Model file for the job. Use its own axes, mm. A direction names the side the tool comes from. Give positions to 0.01 mm unless a question says otherwise; leave off trailing zeros. Write each loop counter-clockwise with the first axis right and the second up, starting at its lowest first coordinate (ties: lowest second). Pieces come first, ordered by that corner, then holes. Notation, with made-up numbers: (30, -14.5) - (81, -14.5) arc R15 cw to (81, 3.5) - close; hole circle Ø8 at (56, 69.25). An arc over 180 degrees is marked (long way). One line per item, written item: value. Start each with the question number.
(1) 3-axis set-ups, long thin cutter, end or side, ignore diameter. For faces 1 (the face through (-3, -3, 11.176)), 2 (the face through (5, 2, 0)): which of +Z, -Z, +X, -X, +Y, -Y reach the whole face in a straight line?
(2) Drop flat-ended pins along their axis: P1, Ø1.5, axis at y = 0.5, z = 9, coming from the -X side; P2, Ø1, axis at y = 2, z = 4, coming from the -X side; P3, Ø2, axis at x = -2.5, z = 10, coming from the +Y side. Give the stop position or say it passes through.
(3) Cut at D-D, the plane z = 2.75. List the corners of the cut face in (x, y), and give its area (3 significant figures).
(4) Cut at C-C, the plane y = -4.75. List the corners of the cut face in (x, z), and give its area (3 significant figures).
(5) Mould opens along Y. For faces 3 (the face through (0.9, -3.9, -0.9)), 4 (the face through (-3, -3, -1.778)), 5 (the face through (-0.661, 5.037, 5.51)), 6 (the face through (-0.86, -3.874, 5.51)) say: pulls with the +Y half, pulls with the -Y half, needs draft (parallel to the pull), parting line crosses it, or undercut.
(6) Probe L1, parallel to Y at x = 0, z = 7; L2, parallel to Y at x = 0, z = -1.1; L3, parallel to Z at x = 4, y = 4.75. List the from-to ranges inside material, lowest first.
from build123d import *

# Parameters (mm, degrees)
SKETCH1_R      = 5.08
SKETCH1_R_2    = 3.96875
EXTRUDE1_DEPTH = 11.176
SKETCH2_R      = 7.112
SKETCH2_R_2    = 4.0005
EXTRUDE2_DEPTH = 1.778


with BuildPart() as part:
    # Sketch1 → Extrude1 (new body)
    with BuildSketch(Plane.XY):
        Circle(SKETCH1_R)
        Circle(SKETCH1_R_2, mode=Mode.SUBTRACT)
    extrude(amount=EXTRUDE1_DEPTH)

    # Sketch2 → Extrude2 (add)
    with BuildSketch(Plane(origin=(0, 0, 0), x_dir=(-1, 0, 0), z_dir=(0, 0, -1))):
        Circle(SKETCH2_R)
        Circle(SKETCH2_R_2, mode=Mode.SUBTRACT)
    extrude(amount=EXTRUDE2_DEPTH)


solid = part.part
Answers follow:
1. face 1: +Z, +X, -X, +Y, -Y
1. face 2: +Z
2. P1: stops at x = -5.08
2. P2: stops at x = -4.85
2. P3: stops at y = 4.85
3. outline: circle Ø10.16 at (0, 0); hole circle Ø7.94 at (0, 0)
3. area: 31.6 mm²
4. outline: (-5.29, -1.78) - (5.29, -1.78) - (5.29, 0) - (1.8, 0) - (1.8, 11.18) - (-1.8, 11.18) - (-1.8, 0) - (-5.29, 0) - close
4. area: 59.1 mm²
5. face 3: undercut
5. face 4: needs draft
5. face 5: parting line crosses it
5. face 6: undercut
6. L1: y = -5.08 to -3.97, 3.97 to 5.08
6. L2: y = -7.11 to -4, 4 to 7.11
6. L3: z = -1.78 to 0
